Here's the drawing with two shaded views (mm, measured from the low corner). I have some questions. A direction names the side the tool comes from. Round coordinates to 2 decimals unless told otherwise and drop trailing zeros. Loops run counter-clockwise (first coordinate to the right, second up) from the corner with the lowest first, then second, coordinate; pieces in that order, holes last.
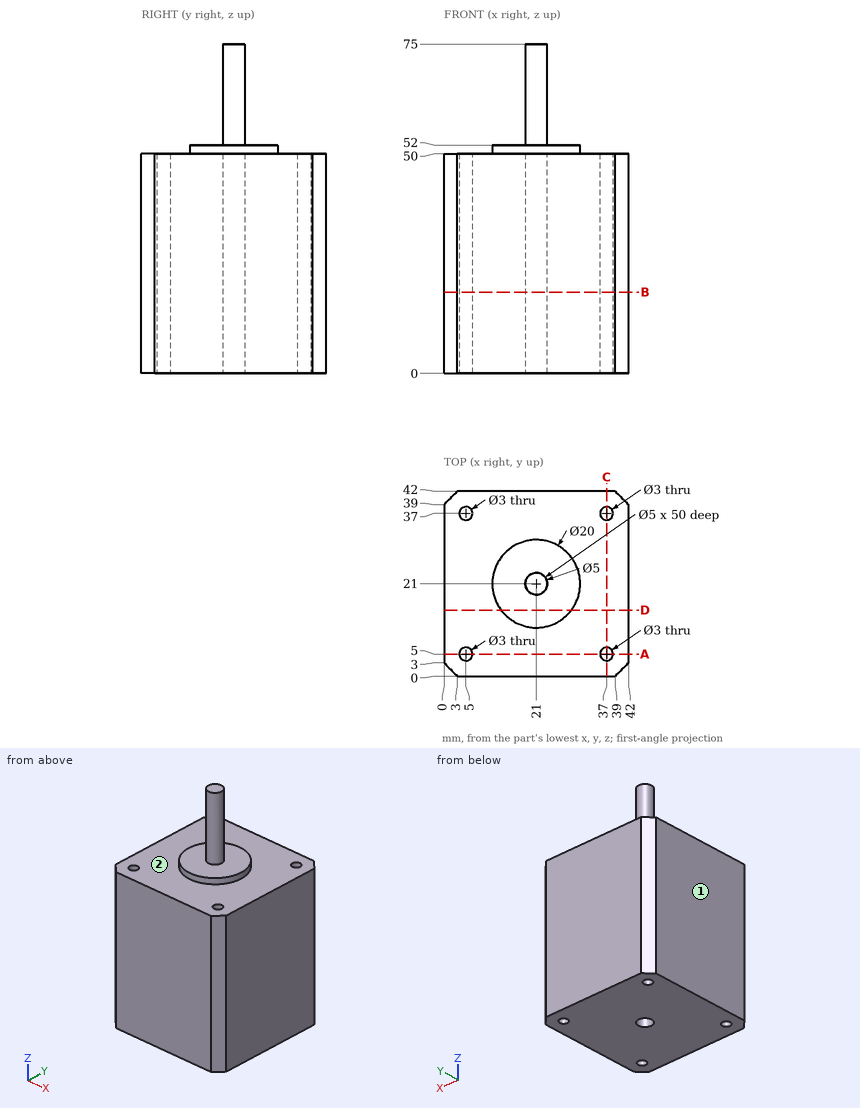
(1) If we section it at D-D, the plane y = 15: List the corners of the cut face in (x, z) for me.
Worked answers:
outline: (0, 0) - (42, 0) - (42, 50) - (29, 50) - (29, 52) - (13, 52) - (13, 50) - (0, 50) - close
(2) If we section it at A-A, the plane y = 5: List the corners of the cut face in (x, z) for me.
Worked answers:
outline: (0, 0) - (3.5, 0) - (3.5, 50) - (0, 50) - close; (6.5, 0) - (35.5, 0) - (35.5, 50) - (6.5, 50) - close; (38.5, 0) - (42, 0) - (42, 50) - (38.5, 50) - close
(3) If I drill on line 1 (Y direction, x = 37, z = 30); line 2 (Y direction, x = 36, z = 44.5), over which ranges is the centre line in solid material (lowest first)?
Worked answers:
line 1: y = 0 to 3.5, 6.5 to 35.5, 38.5 to 42
line 2: y = 0 to 3.88, 6.12 to 35.88, 38.12 to 42
(4) If we section it at B-B, the plane z = 18.5: List the corners of the cut face in (x, y) for me, then the cut area to 3 significant figures.
Worked answers:
outline: (0, 3) - (3, 0) - (39, 0) - (42, 3) - (42, 39) - (39, 42) - (3, 42) - (0, 39) - close; hole circle Ø3 at (5, 5); hole circle Ø3 at (5, 37); hole circle Ø5 at (21, 21); hole circle Ø3 at (37, 5); hole circle Ø3 at (37, 37)
area: 1,700 mm2
(5) Will these pins go through, and if not, where does the flat tip stop? P1, Ø2.5, axis at x = 37, y = 37, coming from the +Z side; P2, Ø4, axis at y = 24, z = 52.5, coming from the +X side; P3, Ø8, axis at x = 21, y = 21, coming from the -Z side; P4, Ø3, axis at x = 35.5, y = 29.5, coming from the +Z side.
Worked answers:
P1: passes through
P2: stops at x = 30.94
P3: stops at z = 0
P4: stops at z = 50
(6) For the marked faces 1 and 2, which set-ups out of +Z, -Z, +X, -X, +Y, -Y let a thin tool reach every point of the face, with its end or its side?
Worked answers:
face 1: +Z, -Z, -X, +Y, -Y
face 2: +Z
